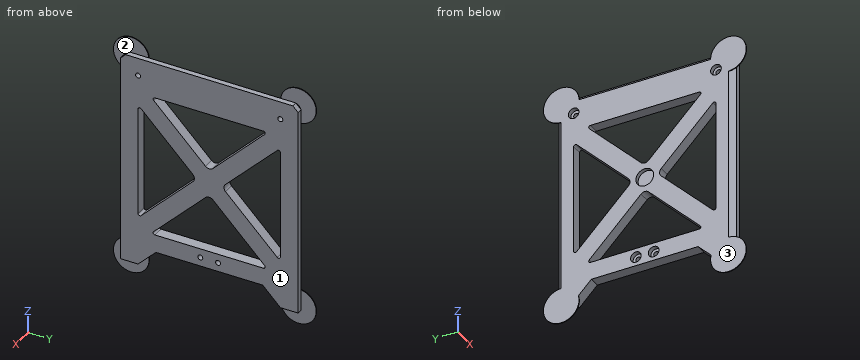
```python
from build123d import *

# Parameters (mm, degrees)
F1_DEPTH       = 6
F2_R           = 1
F3_D           = 2.8
F3_CBORE_D     = 6
F3_CBORE_DEPTH = 2.5
F4_R           = 5
F5_DEPTH       = 2.2
F7_D           = 2.8
F7_CBORE_D     = 6
F7_CBORE_DEPTH = 2.5
F8_SIZE        = 3
F10_DEPTH      = 0.4


with BuildPart() as f1:
    # F0 (on Right) → F1 (new body)
    with BuildSketch(Plane.YZ):
        Polygon((40.0512183458, -60), (50, -60), (50, 60), (-50, 60), (-50, -60), (-40, -60), (-29.9487816542, -50), (30.0512183458, -50), align=None)
        with BuildLine():
            Line((2.1213203436, -9.1923881554), (32.9289321881, -40))
            Line((32.9289321881, -40), (-32.9289321881, -40))
            Line((-32.9289321881, -40), (-2.1213203436, -9.1923881554))
            ThreePointArc((-2.1213203436, -9.1923881554), (0, -8.313708499), (2.1213203436, -9.1923881554))
        make_face(mode=Mode.SUBTRACT)
        with BuildLine():
            Line((-9.1923881554, -2.1213203436), (-40, -32.9289321881))
            Line((-40, -32.9289321881), (-40, 32.9289321881))
            Line((-40, 32.9289321881), (-9.1923881554, 2.1213203436))
            ThreePointArc((-9.1923881554, 2.1213203436), (-8.313708499, 0), (-9.1923881554, -2.1213203436))
        make_face(mode=Mode.SUBTRACT)
        with BuildLine():
            Line((40, 32.9289321881), (40, -32.9289321881))
            Line((40, -32.9289321881), (9.1923881554, -2.1213203436))
            ThreePointArc((9.1923881554, -2.1213203436), (8.313708499, 0), (9.1923881554, 2.1213203436))
            Line((9.1923881554, 2.1213203436), (40, 32.9289321881))
        make_face(mode=Mode.SUBTRACT)
        with BuildLine():
            Line((-32.9289321881, 40), (32.9289321881, 40))
            Line((32.9289321881, 40), (2.1213203436, 9.1923881554))
            ThreePointArc((2.1213203436, 9.1923881554), (0, 8.313708499), (-2.1213203436, 9.1923881554))
            Line((-2.1213203436, 9.1923881554), (-32.9289321881, 40))
        make_face(mode=Mode.SUBTRACT)
    extrude(amount=F1_DEPTH)

    # F2
    f2_edges = [f1.edges().sort_by_distance(p)[0] for p in [
        (3, -32.928932, 40),
        (3, 32.928932, 40),
        (3, -40, 32.928932),
        (3, -40, -32.928932),
        (3, -32.928932, -40),
        (3, 40, 32.928932),
        (3, 40, -32.928932),
        (3, 32.928932, -40),
    ]]
    fillet(f2_edges, radius=F2_R)

    # F3 (through all)
    with Locations(Plane(origin=(0, 0, 0), x_dir=(0, 1, 0), z_dir=(-1, 0, 0))):
        with Locations((-40, -50), (40, -50)):
            CounterBoreHole(F3_D / 2, F3_CBORE_D / 2, F3_CBORE_DEPTH)

    # F4 (on face) → F5 (cut)
    with BuildSketch(Plane(origin=(0, 0, 0), x_dir=(0, -1, 0), z_dir=(-1, 0, 0))):
        Circle(F4_R)
    extrude(amount=-F5_DEPTH, mode=Mode.SUBTRACT)

    # F7 (through all)
    with Locations(Plane(origin=(0, 0, 0), x_dir=(0, -1, 0), z_dir=(-1, 0, 0))):
        with Locations((-5, -45), (5, -45)):
            CounterBoreHole(F7_D / 2, F7_CBORE_D / 2, F7_CBORE_DEPTH)

    # F8
    f8_edges = [f1.edges().sort_by_distance(p)[0] for p in [
        (3, -50, 60),
        (3, 50, 60),
        (0, -50, 0),
        (0, 50, 0),
        (0, 0, 60),
    ]]
    chamfer(f8_edges, length=F8_SIZE)

    # F9 (on face) → F10 (join)
    with BuildSketch(Plane(origin=(0, 0, 0), x_dir=(0, -1, 0), z_dir=(-1, 0, 0))):
        with BuildLine():
            Line((-47, 57), (-37, 57))
            ThreePointArc((-37, 57), (-54.0710678119, 64.0710678119), (-47, 47))
            Line((-47, 47), (-47, 57))
        make_face()
        with BuildLine():
            ThreePointArc((47, 47), (54.0710678119, 64.0710678119), (37, 57))
            Line((37, 57), (47, 57))
            Line((47, 57), (47, 47))
        make_face()
        with BuildLine():
            Line((-47, -60), (-47, -50))
            ThreePointArc((-47, -50), (-53.0480452096, -67.9637396456), (-37.3669885172, -57.3157701715))
            Line((-37.3669885172, -57.3157701715), (-40.0512183458, -60))
            Line((-40.0512183458, -60), (-47, -60))
        make_face()
        with BuildLine():
            ThreePointArc((37.3529996858, -57.3664880981), (53.0689735945, -67.9478021811), (47, -50))
            Line((47, -50), (47, -60))
            Line((47, -60), (40, -60))
            Line((40, -60), (37.3529996858, -57.3664880981))
        make_face()
    extrude(amount=-F10_DEPTH)


solid = f1.part
```
Here's how the part is built. I have some questions about the finished solid (model axes, mm). Face numbers are marked on the shaded views. Coordinates: 2 decimals unless noted, no trailing zeros. Order: outer loops, then holes, each group sorted by start corner. A loop starts at its lowest first (then second) coordinate and runs counter-clockwise, first axis right, second up. Notation, with made-up numbers: (-15, 61) - (7, 61) arc R17 ccw to (7, 68) - close; hole circle Ø11 at (-7, 53.5). An arc over 180 degrees is marked (long way). One line per question, with ' | ' between items. Start each with the question number.
1. If we mould it in two halves opening along X, with no side actions, what happens to the marked faces 1, 2 and 3? For each: released by +X, released by -X, zero draft, split by the parting line, or undercut.
2. If we section it at A-A (z = 0): Write out the boundary of the cut face in (x, y), and give its area (3 significant figures).
3. If we section it at C-C (z = -33): Write out the boundary of the cut face in (x, y).
4. I'm going to push flat-ended pins straight in: pin 1 Ø1.8 at (y, z) = (-39.5, 49) entering from -X; pin 2 Ø1.5 at (x, z) = (5, 17.5) entering from +Y; pin 3 Ø1.7 at (x, y) = (2.5, -43.5) entering from -Z. Where does each tip first touch, or does it pass through?
5. If we section it at B-B (y = -15): Write out the boundary of the cut face in (x, z), and give its area (3 significant figures).
6. If we section it at D-D (x = 4.5): Give the number of separate pieces and of enclosed holes in the cut face, and give its area (3 significant figures).
7. Please list where these lines run through material, in increasing order: line 1 along Y through (x, z) = (1.15, 50); line 2 along Y through (x, z) = (3.3, 50); line 3 along Z through (x, y) = (3.75, -25). Write a range as [from, to].
Model answer:
1) face 1: released by +X | face 2: undercut | face 3: released by -X
2) outline: (0, -47) - (3, -50) - (6, -50) - (6, -40) - (0, -40) - close; (0, -8.31) - (6, -8.31) - (6, 8.31) - (0, 8.31) - (0, 5) - (2.2, 5) - (2.2, -5) - (0, -5) - close; (0, 40) - (6, 40) - (6, 50) - (3, 50) - (0, 47) - close | area: 189 mm²
3) outline: (0, -47) - (3, -50) - (6, -50) - (6, -25.93) - (0, -25.93) - close; (0, 25.93) - (6, 25.93) - (6, 50) - (3, 50) - (0, 47) - close
4) pin 1: stops at x = 2.5 | pin 2: stops at y = 50 | pin 3: stops at z = -60
5) outline: (0, -50) - (6, -50) - (6, -40) - (0, -40) - close; (0, -22.07) - (6, -22.07) - (6, -7.93) - (0, -7.93) - close; (0, 7.93) - (6, 7.93) - (6, 22.07) - (0, 22.07) - close; (0, 40) - (6, 40) - (6, 60) - (3, 60) - (0, 57) - close | area: 345 mm²
6) separate pieces: 1 | enclosed holes: 8 | area: 6,950 mm²
7) line 1: y = [-48.15, -43], [-37, 37], [43, 48.15] | line 2: y = [-50, -41.4], [-38.6, 38.6], [41.4, 50] | line 3: z = [-50, -40], [-32.07, -17.93], [17.93, 32.07], [40, 60]
